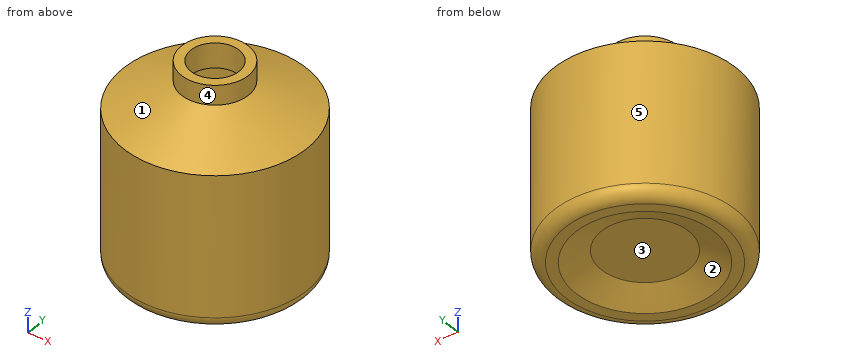
from build123d import *


with BuildPart() as f1:
    # F0 (on Front) → F1 (revolve)
    with BuildSketch(Plane.XZ):
        with BuildLine():
            Line((0, 2.203822), (0, 0))
            Line((0, 0), (14.114344, 0))
            Line((14.114344, 0), (22.420958, -3.83735))
            Line((22.420958, -3.83735), (25.736834, -3.83735))
            ThreePointArc((25.736834, -3.83735), (28.430911, -2.721426), (29.546834, -0.02735))
            Line((29.546834, -0.02735), (29.546834, 45.425702))
            Line((29.546834, 45.425702), (10.819199, 54.336432))
            Line((10.819199, 54.336432), (10.819199, 60.679659))
            Line((10.819199, 60.679659), (7.798612, 60.679659))
            Line((7.798612, 60.679659), (7.798612, 52.675109))
            Line((7.798612, 52.675109), (26.677277, 43.31129))
            Line((26.677277, 43.31129), (26.677277, 2.540149))
            ThreePointArc((26.677277, 2.540149), (25.561354, -0.153928), (22.867277, -1.269851))
            Line((22.867277, -1.269851), (22.118898, -1.269851))
            Line((22.118898, -1.269851), (15.775668, 2.203822))
            Line((15.775668, 2.203822), (0, 2.203822))
        make_face()
    revolve(axis=Axis((0, 0, 30.669179), (0, 0, 1)))


solid = f1.part
Geometry check sheet. Reference: the model listing, model coordinates, mm. Face numbers are marked on the shaded views. A direction names the side the tool comes from. Round coordinates to 2 decimals unless told otherwise and drop trailing zeros. Write each loop counter-clockwise with the first axis right and the second up, starting at its lowest first coordinate (ties: lowest second). Pieces come first, ordered by that corner, then holes. Notation, with made-up numbers: (-20.75, 38.5) - (37.25, 38.5) arc R18 cw to (37.25, 43.5) - close; hole circle Ø4 at (-22.75, 35.5). An arc over 180 degrees is marked (long way). One line per item, written item: value.
1. Scan lines: L1, parallel to Y at x = 0, z = 24.5; L2, parallel to Y at x = 0, z = 57; L3, parallel to Y at x = -7.5, z = -0.5. Record each from-to range of solid material in increasing order.
The answers:
L1: y = -29.55 to -26.68, 26.68 to 29.55
L2: y = -10.82 to -7.8, 7.8 to 10.82
L3: y = -28.55 to -24.02, -19.31 to -13.22, 13.22 to 19.31, 24.02 to 28.55
2. Cross-section at A-A on y = 0. Record the boundary of the cut face in (x, z).
The answers:
outline: (-29.55, -0.03) arc R3.81 ccw to (-25.74, -3.84) - (-22.42, -3.84) - (-14.11, 0) - (14.11, 0) - (22.42, -3.84) - (25.74, -3.84) arc R3.81 ccw to (29.55, -0.03) - (29.55, 45.43) - (10.82, 54.34) - (10.82, 60.68) - (7.8, 60.68) - (7.8, 52.68) - (26.68, 43.31) - (26.68, 2.54) arc R3.81 cw to (22.87, -1.27) - (22.12, -1.27) - (15.78, 2.2) - (-15.78, 2.2) - (-22.12, -1.27) - (-22.87, -1.27) arc R3.81 cw to (-26.68, 2.54) - (-26.68, 43.31) - (-7.8, 52.68) - (-7.8, 60.68) - (-10.82, 60.68) - (-10.82, 54.34) - (-29.55, 45.43) - close
3. Depth check by flat-ended pin: pin 1 Ø2 at (y, z) = (17.5, 53.5) entering from +X; pin 2 Ø10 at (y, z) = (11.5, 26.5) entering from +X; pin 3 Ø3 at (x, z) = (7, 23) entering from +Y; pin 4 Ø3 at (y, z) = (23, 26) entering from -X. Enter the tip coordinate at first touch or a pass-through.
The answers:
pin 1: passes through
pin 2: stops at x = 28.82
pin 3: stops at y = 29.03
pin 4: stops at x = -20.27
4. Set-up check for the marked faces 3, 4 and 5: record each of +Z, -Z, +X, -X, +Y, -Y from which the full face is reachable in a straight line by a thin tool's end or side.
The answers:
face 3: -Z
face 4: +Z
face 5: +Z, -Z
5. Cross-section at C-C on z = 1. Record the boundary of the cut face in (x, y).
The answers:
outline: circle Ø59.09 at (0, 0); circle Ø35.95 at (0, 0); hole circle Ø52.7 at (0, 0)
6. Mould release check, pull along X, two halves, no side actions. Record for the marked faces 1 and 2: released by +X, released by -X, zero draft, split by the parting line, or undercut.
The answers:
face 1: split by the parting line
face 2: undercut
7. Cross-section at D-D on z = 37.5. Record the boundary of the cut face in (x, y), and give its area (3 significant figures).
The answers:
outline: circle Ø59.09 at (0, 0); hole circle Ø53.35 at (0, 0)
area: 507 mm^2
